Autodesk Inventor part; units mm, degrees
ref_plane "YZ Plane" through (0, 0, 0) normal (1, 0, 0) x (0, 1, 0)
ref_plane "XZ Plane" through (0, 0, 0) normal (0, 1, 0) x (-1, 0, 0)
ref_plane "XY Plane" through (0, 0, 0) normal (0, 0, 1) x (1, 0, 0)
sketch "Base" plane through (0, 0, 0) normal (0, 0, 1) x (1, 0, 0)
  line L0 (-22, -39.56) -> (22, -39.56)
  line L1 (22, -39.56) -> (22, 39.56)
  line L2 (22, 39.56) -> (-22, 39.56)
  line L3 (-22, 39.56) -> (-22, -39.56)
  line L4 (-22, -39.56) -> (22, 39.56) construction
  line L5 (22, -39.56) -> (-22, 39.56) construction
  point P0 (0, 0)
  dimension "d56" = 44
  dimension "d57" = 79
extrude "Extrusion4" add sketch "Base" along normal blind 6
sketch "Slot1" plane through (0, 0, 6) normal (0, 0, 1) x (1, 0, 0)
  line L0 (21, -38.56) -> (-21, -38.56)
  line L1 (-21, -38.56) -> (-21, -30.44)
  line L2 (-21, -30.44) -> (21, -30.44)
  line L3 (21, -30.44) -> (21, -38.56)
  line L4 (21, -38.56) -> (-21, -30.44) construction
  line L5 (-21, -38.56) -> (21, -30.44) construction
  line L6 (22, -39.56) -> (22, 39.56)
  line L7 (-22, -39.56) -> (22, -39.56)
  point P0 (0, 0)
  point P1 (0, -34.5)
  dimension "d62" = 8.1
  dimension "d63" = 1
  dimension "d64" = 42
  dimension "d66" = 1
extrude "Slot1 slot" cut sketch "Slot1" against normal blind 4
sketch "Slot2" plane through (0, 0, 6) normal (0, 0, 1) x (1, 0, 0)
  line L0 (21, -0.44) -> (-21, -0.44)
  line L1 (-21, -0.44) -> (-21, 6.08)
  line L2 (-21, 6.08) -> (21, 6.08)
  line L3 (21, 6.08) -> (21, -0.44)
  line L4 (21, -0.44) -> (-21, 6.08) construction
  line L5 (-21, -0.44) -> (21, 6.08) construction
  line L6 (-22, 39.56) -> (-22, -39.56)
  line L7 (-21, -30.44) -> (21, -30.44)
  point P0 (0, 0)
  point P1 (0, 2.82)
  dimension "d75" = 6.5
  dimension "d76" = 42
  dimension "d77" = 1
  dimension "d80" = 30
extrude "Slot2 slot" cut sketch "Slot2" against normal blind 4
sketch "Slot3" plane through (0, 0, 6) normal (0, 0, 1) x (1, 0, 0)
  line L0 (-21, 38.2) -> (21, 38.2)
  line L1 (21, 38.2) -> (21, 34.08)
  line L2 (21, 34.08) -> (-21, 34.08)
  line L3 (-21, 34.08) -> (-21, 38.2)
  line L4 (-21, 38.2) -> (21, 34.08) construction
  line L5 (21, 38.2) -> (-21, 34.08) construction
  point P0 (0, 36.14)
  dimension "d83" = 4.1
  dimension "d84" = 42
extrude "Extrusion7" cut sketch "Slot3" against normal blind 4
fillet "Fillet1" radius 2 1 edges at (-22, 39.56, 3)
fillet "Fillet2" radius 2 1 edges at (22, 39.56, 3)
fillet "Fillet3" radius 2 1 edges at (22, -39.56, 3)
fillet "Fillet4" radius 2 1 edges at (-22, -39.56, 3)
sketch "Sketch14" plane through (0, 0, 6) normal (0, 0, 1) x (1, 0, 0)
  arc A0 (-22, -37.56) -> (-20, -39.56) centre (-20, -37.56) ccw
  line L0 (-20, -39.56) -> (20, -39.56)
  arc A1 (20, -39.56) -> (22, -37.56) centre (20, -37.56) ccw
  line L1 (22, -37.56) -> (22, 37.56)
  arc A2 (22, 37.56) -> (20, 39.56) centre (20, 37.56) ccw
  line L2 (20, 39.56) -> (-20, 39.56)
  arc A3 (-20, 39.56) -> (-22, 37.56) centre (-20, 37.56) ccw
  line L3 (-22, 37.56) -> (-22, -37.56)
  line L4 (-21, 34.08) -> (-21, 38.2)
  line L5 (-21, 38.2) -> (21, 38.2)
  line L6 (21, 38.2) -> (21, 34.08)
  line L7 (21, 34.08) -> (-21, 34.08)
  line L8 (21, 6.08) -> (21, -0.44)
  line L9 (21, -0.44) -> (-21, -0.44)
  line L10 (-21, -0.44) -> (-21, 6.08)
  line L11 (-21, 6.08) -> (21, 6.08)
  line L12 (21, -30.44) -> (21, -38.56)
  line L13 (21, -38.56) -> (-21, -38.56)
  line L14 (-21, -38.56) -> (-21, -30.44)
  line L15 (-21, -30.44) -> (21, -30.44)
  line L16 (20, 39.56) -> (-20, 39.56)
  line L17 (-20, 39.56) -> (-20, 38.2)
  line L18 (-20, 38.2) -> (20, 38.2)
  line L19 (20, 38.2) -> (20, 39.56)
  line L20 (-21, 38.2) -> (21, 38.2)
  line L21 (-21, 34.08) -> (21, 34.08)
  line L22 (21, 34.08) -> (21, 31.08)
  line L23 (21, 31.08) -> (-21, 31.08)
  line L24 (-21, 31.08) -> (-21, 34.08)
  line L25 (-21, 6.08) -> (21, 6.08)
  line L26 (21, 6.08) -> (21, 9.08)
  line L27 (21, 9.08) -> (-21, 9.08)
  line L28 (-21, 9.08) -> (-21, 6.08)
  line L29 (-21, -0.44) -> (21, -0.44)
  line L30 (21, -0.44) -> (21, -3.44)
  line L31 (21, -3.44) -> (-21, -3.44)
  line L32 (-21, -3.44) -> (-21, -0.44)
  dimension "d95" = 3
extrude "Extrusion9" add sketch "Sketch14" along normal blind 5 contours L2 L19 L5 L17 | L7 L22 L23 L24 | L11 L28 L27 L26 | L30 L31 L32 L9
equation "\"d56\" = basew"
equation "\"d57\" = baseh"
equation "\"d62\" = wall1slot"
equation "\"d63\" = -0.5 * wallw + 0.5 * basew"
equation "\"d64\" = wallw"
equation "\"d66\" = 0.5 * baseextra"
equation "\"d75\" = wall2slot"
equation "\"d76\" = wallw"
equation "\"d77\" = 0.5 * baseextra"
equation "\"d80\" = gap1"
equation "\"d83\" = wall3slot"
equation "\"d84\" = wallw"
equation "\"printer3dtolerance\" = 0.1"
equation "\"wallw\" = 42"
equation "\"wallh\" = 44"
equation "\"cornerrad\" = 2"
equation "\"baseextra\" = 2"
equation "\"wall1_thick\" = 8"
equation "\"wall2_thick\" = 6.4"
equation "\"wall3_thick\" = 4"
equation "\"wall1slot\" = 8.1"
equation "\"wall2slot\" = 6.5"
equation "\"wall3slot\" = 4.1"
equation "\"gap1\" = 30"
equation "\"gap2\" = 28"
equation "\"baseh\" = 79"
equation "\"basew\" = 44"
equation "\"base_thick\" = 6"
equation "\"base_slots_depth\" = 4"
equation "\"d26\" = 8.12"
equation "\"d27\" = 42"
equation "\"d28\" = 44"
equation "\"d29\" = 28"
equation "\"d31\" = 4.12"
equation "\"d32\" = 6.52"
equation "\"d33\" = 79.12"
equation "\"d39\" = 8.12"
equation "\"d40\" = 42"
equation "\"d41\" = 44"
equation "\"d48\" = 8.12"
equation "\"d49\" = 42"
equation "\"d50\" = 8.12"
equation "\"d51\" = 42"
equation "\"d52\" = 44"
equation "\"d53\" = 44"
equation "\"d71\" = 8.12"
equation "\"d72\" = 42"
equation "\"d73\" = 2"
equation "\"d74\" = 44"
equation "\"distancefrombottom\" = 34"
equation "\"servosmallcircledia\" = 5.9"
equation "\"servo9gw\" = 22.8"
equation "\"servomountsquare\" = 4"
equation "\"servopolygonl\" = 5.9"
equation "\"servopolygonr\" = 6.1"
equation "\"distancefromleft\" = 22"
equation "\"servobigcircledia\" = 11.6"
equation "\"servomounth\" = 4"
equation "\"wall3slotd\" = 2"
equation "\"wall3slotw\" = 36"
equation "\"adapterh\" = 16"
equation "\"adapterw\" = 32"
equation "\"wall3slotd_1\" = 2"
equation "\"armslotd\" = 2"
equation "\"armthick\" = 3"
equation "\"armw\" = 34"
equation "\"fanhs\" = 9.6"
equation "\"fanhb\" = 11"
equation "\"adapterwallslotd\" = 2"
equation "\"adapterwallthick\" = 6"
equation "\"hornscrewholed\" = 2"
equation "\"hornscrewheadd\" = 3"
equation "\"armhornthick\" = 3"
equation "\"hornthick\" = 1.5"
properties part number "base-frame" material "Wood (Oak)"
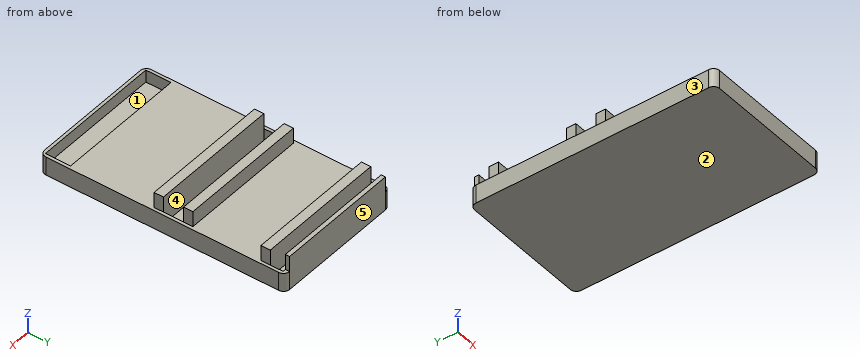
Check sheet for the modelled part. Datum: model origin and axes. Units: mm. Face numbers are marked on the shaded views. A direction names the side the tool comes from. Round coordinates to 2 decimals unless told otherwise and drop trailing zeros. Order: outer loops, then holes, each group sorted by start corner. A loop starts at its lowest first (then second) coordinate and runs counter-clockwise, first axis right, second up.
(1) Cross-section at B-B, the plane z = 3.5. Enter the section's corners in (x, y), and give its area (3 significant figures).
(2) Cross-section at C-C, the plane x = 1.5. Enter the section's corners in (y, z), and give its area (3 significant figures).
(3) Scan lines: probe 1 along Y at (x, z) = (18, 9); probe 2 along Y at (x, z) = (20.5, 6.5); probe 3 along Y at (x, z) = (9, 5.5). Record each from-to range of solid material in increasing order.
(4) Go/stop test with flat-tipped pins: P1, Ø1, axis at x = -3, y = -27.5, coming from the -Z side; P2, Ø2.5, axis at y = 32.5, z = 9, coming from the -X side; P3, Ø1.5, axis at y = 32, z = 8, coming from the +X side; P4, Ø4, axis at x = -8, y = -36.5, coming from the +Z side. Record where each tip stops, or that it passes through.
(5) Cross-section at D-D, the plane y = -2. Enter the section's corners in (x, z).
(6) Access from +Z, -Z, +X, -X, +Y, -Y to the whole of each face (thin tool, end or side, straight path). Record for the marked faces 1 and 2.
(7) Draft check along Y on the marked faces 3, 4 and 5. Enter one of: pulls with the +Y half, pulls with the -Y half, needs draft (parallel to the pull), parting line crosses it, or undercut.
(8) Cross-section at A-A, the plane z = 10.25. Enter the section's corners in (x, y), and give its area (3 significant figures).
Check sheet entries:
1. outline: (-22, -37.56) arc R2 ccw to (-20, -39.56) - (20, -39.56) arc R2 ccw to (22, -37.56) - (22, 37.56) arc R2 ccw to (20, 39.56) - (-20, 39.56) arc R2 ccw to (-22, 37.56) - close; hole (-21, -38.56) - (21, -38.56) - (21, -30.44) - (-21, -30.44) - close; hole (-21, -0.44) - (21, -0.44) - (21, 6.08) - (-21, 6.08) - close; hole (-21, 34.08) - (21, 34.08) - (21, 38.2) - (-21, 38.2) - close
1. area: 2,690 mm2
2. outline: (-39.56, 0) - (39.56, 0) - (39.56, 11) - (38.2, 11) - (38.2, 2) - (34.08, 2) - (34.08, 11) - (31.08, 11) - (31.08, 6) - (9.08, 6) - (9.08, 11) - (6.08, 11) - (6.08, 2) - (-0.44, 2) - (-0.44, 11) - (-3.44, 11) - (-3.44, 6) - (-30.44, 6) - (-30.44, 2) - (-38.56, 2) - (-38.56, 6) - (-39.56, 6) - close
2. area: 451 mm2
3. probe 1: y = -3.44 to -0.44, 6.08 to 9.08, 31.08 to 34.08, 38.2 to 39.56
3. probe 2: y = -3.44 to -0.44, 6.08 to 9.08, 31.08 to 34.08
3. probe 3: y = -39.56 to -38.56, -30.44 to -0.44, 6.08 to 34.08, 38.2 to 39.56
4. P1: stops at z = 0
4. P2: stops at x = -21
4. P3: stops at x = 21
4. P4: stops at z = 2
5. outline: (-22, 0) - (22, 0) - (22, 6) - (21, 6) - (21, 11) - (-21, 11) - (-21, 6) - (-22, 6) - close
6. face 1: +Z
6. face 2: -Z, +X, -X, +Y, -Y
7. face 3: needs draft
7. face 4: undercut
7. face 5: pulls with the +Y half
8. outline: (-21, -3.44) - (21, -3.44) - (21, -0.44) - (-21, -0.44) - close; (-21, 6.08) - (21, 6.08) - (21, 9.08) - (-21, 9.08) - close; (-21, 31.08) - (21, 31.08) - (21, 34.08) - (-21, 34.08) - close; (-20, 38.2) - (20, 38.2) - (20, 39.56) - (-20, 39.56) - close
8. area: 432 mm2
